The listing builds one solid part. Answer for the finished solid, in the listing's coordinates (mm). Face numbers are marked on the shaded views. A direction names the side the tool comes from. Coordinates: 2 decimals unless noted, no trailing zeros. Loops run counter-clockwise (first coordinate to the right, second up) from the corner with the lowest first, then second, coordinate; pieces in that order, holes last. Notation, with made-up numbers: (8.25, 68.5) -> (64.25, 68.5) arc R29 cw to (64.25, 88.5) -> close; hole circle Ø4 at (37.25, 33.25). An arc over 180 degrees is marked (long way). Answer in a Markdown table with one row per item.
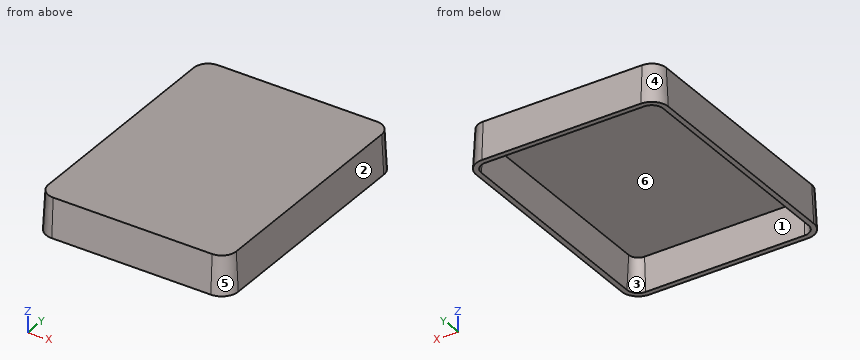
```python
from build123d import *

# Parameters (mm, degrees)
F1_DEPTH = 15
F1_TAPER = 3
F2_T     = -2


with BuildPart() as f1:
    # F0 (on Top) → F1 (new body)
    with BuildSketch(Plane.XY):
        with BuildLine():
            ThreePointArc((36.9276963174, 42.0978697181), (35.067824378, 46.5879977786), (30.5776963174, 48.4478697181))
            Line((30.5776963174, 48.4478697181), (-30.5776963174, 48.4478697181))
            ThreePointArc((-30.5776963174, 48.4478697181), (-35.067824378, 46.5879977786), (-36.9276963174, 42.0978697181))
            Line((-36.9276963174, 42.0978697181), (-36.9276963174, -42.0978697181))
            ThreePointArc((-36.9276963174, -42.0978697181), (-35.067824378, -46.5879977786), (-30.5776963174, -48.4478697181))
            Line((-30.5776963174, -48.4478697181), (30.5776963174, -48.4478697181))
            ThreePointArc((30.5776963174, -48.4478697181), (35.067824378, -46.5879977786), (36.9276963174, -42.0978697181))
            Line((36.9276963174, -42.0978697181), (36.9276963174, 42.0978697181))
        make_face()
    extrude(amount=F1_DEPTH, taper=F1_TAPER)

    # F2
    f2_openings = [f1.faces().sort_by_distance(p)[0] for p in [
        (0, 0, 0),
    ]]
    offset(amount=F2_T, openings=f2_openings)


solid = f1.part
```
Item 1: A cutting plane is placed at A-A, the plane x = -26. Determine the outline of the cut face in (y, z), plus the area to 3 significant figures.
Findings below:
| item | result |
|---|---|
| outline | (-48.45, 0) -> (-46.45, 0) -> (-45.76, 13) -> (45.76, 13) -> (46.45, 0) -> (48.45, 0) -> (47.66, 15) -> (-47.66, 15) -> close |
| area | 243 mm2 |
Item 2: Find the intervals of material crossed by probe 1 along Z at (x, y) = (-18.5, -38.5); probe 2 along Y at (x, z) = (-20, 6); probe 3 along X at (y, z) = (17.5, 9), in increasing order.
Findings below:
| item | result |
|---|---|
| probe 1 | z = 13 to 15 |
| probe 2 | y = -48.13 to -46.13, 46.13 to 48.13 |
| probe 3 | x = -36.46 to -34.45, 34.45 to 36.46 |
Item 3: Determine the mould class of the marked faces 3, 4, 5 and 6 for opening direction Y: +Y half, -Y half, draft (parallel to the pull), parting line (faces both ways), or undercut.
Findings below:
| item | result |
|---|---|
| face 3 | undercut |
| face 4 | +Y half |
| face 5 | -Y half |
| face 6 | undercut |
Item 4: A cutting plane is placed at B-B, the plane y = -38.5. Determine the outline of the cut face in (x, z).
Findings below:
| item | result |
|---|---|
| outline | (-36.93, 0) -> (-34.92, 0) -> (-34.24, 13) -> (34.24, 13) -> (34.92, 0) -> (36.93, 0) -> (36.14, 15) -> (-36.14, 15) -> close |
Item 5: A cutting plane is placed at D-D, the plane z = 6. Determine the outline of the cut face in (x, y).
Findings below:
| item | result |
|---|---|
| outline | (-36.61, -42.1) arc R6.04 ccw to (-30.58, -48.13) -> (30.58, -48.13) arc R6.04 ccw to (36.61, -42.1) -> (36.61, 42.1) arc R6.04 ccw to (30.58, 48.13) -> (-30.58, 48.13) arc R6.04 ccw to (-36.61, 42.1) -> close; hole (-34.61, -42.1) arc R4.03 ccw to (-30.58, -46.13) -> (30.58, -46.13) arc R4.03 ccw to (34.61, -42.1) -> (34.61, 42.1) arc R4.03 ccw to (30.58, 46.13) -> (-30.58, 46.13) arc R4.03 ccw to (-34.61, 42.1) -> close |
Item 6: A cutting plane is placed at C-C, the plane z = 11. Determine the outline of the cut face in (x, y).
Findings below:
| item | result |
|---|---|
| outline | (-36.35, -42.1) arc R5.77 ccw to (-30.58, -47.87) -> (30.58, -47.87) arc R5.77 ccw to (36.35, -42.1) -> (36.35, 42.1) arc R5.77 ccw to (30.58, 47.87) -> (-30.58, 47.87) arc R5.77 ccw to (-36.35, 42.1) -> close; hole (-34.35, -42.1) arc R3.77 ccw to (-30.58, -45.87) -> (30.58, -45.87) arc R3.77 ccw to (34.35, -42.1) -> (34.35, 42.1) arc R3.77 ccw to (30.58, 45.87) -> (-30.58, 45.87) arc R3.77 ccw to (-34.35, 42.1) -> close |
Item 7: A tool of negligible diameter and unlimited length cuts with its end or side. For the marked faces 1 and 2, from which of +Z, -Z, +X, -X, +Y, -Y can it reach the whole face along a straight path? Write none if from no direction.
Findings below:
| item | result |
|---|---|
| face 1 | -Z |
| face 2 | +Z, +X, +Y, -Y |
Item 8: Flat-ended cylindrical pins translate along their axes: pin 1 Ø1 at (x, y) = (8, -13) entering from -Z; pin 2 Ø8 at (x, z) = (-19, 11.5) entering from -Y; pin 3 Ø5 at (y, z) = (38.5, 11.5) entering from +X. Find the tip coordinate at first contact, or state that the pin passes through.
Findings below:
| item | result |
|---|---|
| pin 1 | stops at z = 13 |
| pin 2 | stops at y = -48.05 |
| pin 3 | stops at x = 36.46 |
